```python
from build123d import *

# Parameters (mm, degrees)
CROQUIS1_W              = 19
CROQUIS1_H              = 16
SALIENTE_EXTRUIR1_DEPTH = 18
CROQUIS2_R              = 0.35
SALIENTE_EXTRUIR2_DEPTH = 4


with BuildPart() as part:
    # Croquis1 → Saliente-Extruir1 (new body)
    with BuildSketch(Plane(origin=(0, 0, 0), x_dir=(1, 0, 0), z_dir=(0, 1, 0))):
        Rectangle(CROQUIS1_W, CROQUIS1_H)
    extrude(amount=SALIENTE_EXTRUIR1_DEPTH)

    # Croquis2 → Saliente-Extruir2 (add)
    with BuildSketch(Plane.XZ):
        with Locations((-5.08, 6.35)):
            Circle(CROQUIS2_R)
        with Locations((5.08, 6.35)):
            Circle(CROQUIS2_R)
        with Locations((5.08, -6.35)):
            Circle(CROQUIS2_R)
        with Locations((-5.08, -6.35)):
            Circle(CROQUIS2_R)
    extrude(amount=SALIENTE_EXTRUIR2_DEPTH)


solid = part.part
```
Can you work these out from the model? Positions are in its coordinate system, mm. Round coordinates to 2 decimals unless told otherwise and drop trailing zeros. Order: outer loops, then holes, each group sorted by start corner. A loop starts at its lowest first (then second) coordinate and runs counter-clockwise, first axis right, second up. Notation, with made-up numbers: (-34, 1.5) -> (8, 1.5) arc R6 cw to (8, 10.5) -> close; hole circle Ø11 at (-32, -23.5). An arc over 180 degrees is marked (long way). Return JSON: item names as keys, results as strings. Group by question number.
1. I need wall thicknesses on line 1 (Y direction, x = 5.25, z = -2); line 2 (Z direction, x = -5.25, y = -2). Which ranges of each line are inside material? Lowest first, please. Write a range as [from, to].
2. Will this pin go through, and if not, where does the flat tip stop? pin 1 (1.5 mm diameter, centred on y = -1.5, z = 5.5, fed in from -X).
3. If we section it at B-B, the plane x = -5.08: Write out the boundary of the cut face in (y, z), then the cut area to 3 significant figures.
4. If we section it at C-C, the plane z = 1.5: Write out the boundary of the cut face in (x, y).
5. If we section it at A-A, the plane z = -6.35: Write out the boundary of the cut face in (x, y), then the cut area to 3 significant figures.
Output values:
{
 "1": {"line 1": "[0, 18]", "line 2": "[-6.66, -6.04], [6.04, 6.66]"},
 "2": {"pin 1": "x = -5.42"},
 "3": {"outline": "(-4, -6.7) -> (0, -6.7) -> (0, -8) -> (18, -8) -> (18, 8) -> (0, 8) -> (0, 6.7) -> (-4, 6.7) -> (-4, 6) -> (0, 6) -> (0, -6) -> (-4, -6) -> close", "area": "294 mm²"},
 "4": {"outline": "(-9.5, 0) -> (9.5, 0) -> (9.5, 18) -> (-9.5, 18) -> close"},
 "5": {"outline": "(-9.5, 0) -> (-5.43, 0) -> (-5.43, -4) -> (-4.73, -4) -> (-4.73, 0) -> (4.73, 0) -> (4.73, -4) -> (5.43, -4) -> (5.43, 0) -> (9.5, 0) -> (9.5, 18) -> (-9.5, 18) -> close", "area": "348 mm²"}
}
